```python
from build123d import *

# Parameters (mm, degrees)
F0_W     = 279.4
F0_H     = 76.2
F1_DEPTH = 152.4
F3_DEPTH = 125.1016873866
F4_SIZE2 = 50.8
F4_SIZE  = 101.6
F5_R     = 38.1
F6_DEPTH = 200.5284074694


with BuildPart() as f1:
    # F0 (on Front) → F1 (new body)
    with BuildSketch(Plane.XZ):
        Rectangle(F0_W, F0_H)
    extrude(amount=F1_DEPTH)

    # F2 (on face) → F3 (cut)
    with BuildSketch(Plane.XY.offset(38.1)):
        Polygon((139.7, -152.4), (139.7, -50.8), (12.7, -152.4), align=None)
    extrude(amount=-F3_DEPTH, mode=Mode.SUBTRACT)

    # F4
    f4_edges = [f1.edges().sort_by_distance(p)[0] for p in [
        (139.7, -25.4, 38.1),
    ]]
    f4_side = f1.faces().sort_by_distance((-17.386905, -68.640476, 38.1))[0]
    chamfer(f4_edges, length=F4_SIZE, length2=F4_SIZE2, reference=f4_side)

    # F5 (on face) → F6 (cut)
    with BuildSketch(Plane.XY.offset(38.1)):
        with Locations((-63.5, -76.2)):
            Circle(F5_R)
    extrude(amount=-F6_DEPTH, mode=Mode.SUBTRACT)


solid = f1.part
```
Geometry check sheet. Reference: the model listing, model coordinates, mm. Round coordinates to 2 decimals unless told otherwise and drop trailing zeros. Order: outer loops, then holes, each group sorted by start corner. A loop starts at its lowest first (then second) coordinate and runs counter-clockwise, first axis right, second up. Notation, with made-up numbers: (-25.5, 28.5) -> (30.5, 28.5) arc R21 cw to (30.5, 46.5) -> close; hole circle Ø3 at (56, 81.25). An arc over 180 degrees is marked (long way). Return JSON: item names as keys, results as strings. Group by question number.
Q1. Section check A-A, the plane x = -63.5. Record the boundary of the cut face in (y, z).
Q2. Gauge pin test, flat ends, axial feed: pin 1 (10 mm diameter, centred on x = 36, z = 17, fed in from -Y); pin 2 (2 mm diameter, centred on y = -23, z = 2, fed in from +X); pin 3 (12 mm diameter, centred on x = 96.5, z = -13.5, fed in from -Y). Record the tip position at first contact, or that the pin passes through.
Q3. Section check D-D, the plane y = -12.5. Record the boundary of the cut face in (x, z).
Q4. Section check C-C, the plane y = -103.5. Record the boundary of the cut face in (x, z) (1 decimal).
Q5. Material ranges on probe 1 along Y at (x, z) = (-63.5, 21); probe 2 along Y at (x, z) = (-43.5, -31.5); probe 3 along X at (y, z) = (-76, -8), recorded low to high. Write a range as from..to.
Q6. Release check for a two-part mould opening along Y. For faces 1 (the flat face through (-2, 0, 1)), 2 (the cylindrical face through (-27.16, -64.76, 0.53)), 3 (the flat face through (78.3, -50.4, 18)) record: released by +Y, released by -Y, zero draft, split by the parting line, or undercut.
Q7. Section check B-B, the plane z = -26. Record the boundary of the cut face in (x, y), plus the area to 3 significant figures.
Numbers:
{
 "1": {"outline": "(-152.4, -38.1) -> (-114.3, -38.1) -> (-114.3, 38.1) -> (-152.4, 38.1) -> close; (-38.1, -38.1) -> (0, -38.1) -> (0, 38.1) -> (-38.1, 38.1) -> close"},
 "2": {"pin 1": "y = -137.76", "pin 2": "x = 112.3", "pin 3": "y = -90.16"},
 "3": {"outline": "(-139.7, -38.1) -> (139.7, -38.1) -> (139.7, -12.7) -> (38.1, 38.1) -> (-139.7, 38.1) -> close"},
 "4": {"outline": "(-139.7, -38.1) -> (-90.1, -38.1) -> (-90.1, 38.1) -> (-139.7, 38.1) -> close; (-36.9, -38.1) -> (73.8, -38.1) -> (73.8, 20.2) -> (38.1, 38.1) -> (-36.9, 38.1) -> close"},
 "5": {"probe 1": "-152.4..-114.3, -38.1..0", "probe 2": "-152.4..-108.63, -43.77..0", "probe 3": "-139.7..-101.6, -25.4..108.2"},
 "6": {"face 1": "released by +Y", "face 2": "undercut", "face 3": "zero draft"},
 "7": {"outline": "(-139.7, -152.4) -> (12.7, -152.4) -> (139.7, -50.8) -> (139.7, 0) -> (-139.7, 0) -> close; hole circle Ø76.2 at (-63.5, -76.2)", "area": "31,600 mm^2"}
}
